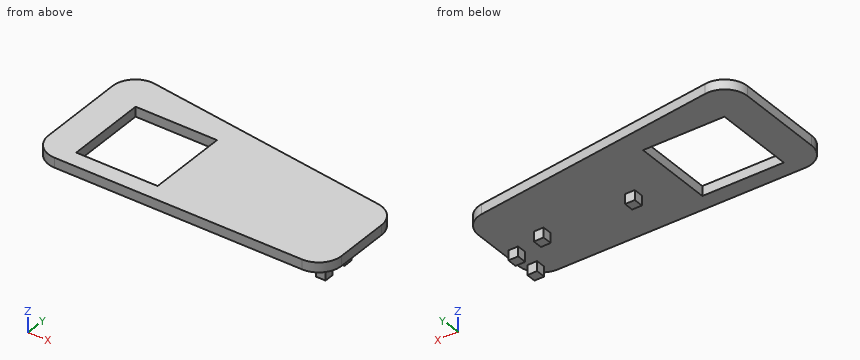
from build123d import *

# Parameters (mm, degrees)
PAD_DEPTH    = 3
SKETCH001_W  = 3
SKETCH001_H  = 3
PAD001_DEPTH = 3
FILLET_R     = 7
SKETCH002_W  = 25
SKETCH002_H  = 25
POCKET_DEPTH = 5


with BuildPart() as part:
    # Sketch → Pad (new body)
    with BuildSketch(Plane.XY):
        Polygon((0, 42), (0, 0), (90, 0), (90, 30), align=None)
    extrude(amount=PAD_DEPTH)

    # Sketch001 (on Face5 of Pad) → Pad001 (join)
    with BuildSketch(Plane(origin=(0, 0, 0), x_dir=(1, 0, 0), z_dir=(0, 0, -1))):
        with Locations((86.5, -4.5)):
            Rectangle(SKETCH001_W, SKETCH001_H)
        with Locations((86.5, -12.5)):
            Rectangle(SKETCH001_W, SKETCH001_H)
        with Locations((76.5, -15.5)):
            Rectangle(SKETCH001_W, SKETCH001_H)
        with Locations((48.5, -15.5)):
            Rectangle(SKETCH001_W, SKETCH001_H)
    extrude(amount=PAD001_DEPTH)

    # Fillet
    fillet_edges = [part.edges().sort_by_distance(p)[0] for p in [
        (0, 42, 1.5),
        (0, 0, 1.5),
        (90, 0, 1.5),
        (90, 30, 1.5),
    ]]
    fillet(fillet_edges, radius=FILLET_R)

    # Sketch002 (on Face2 of Fillet) → Pocket (cut)
    with BuildSketch(Plane(origin=(0, 0, 0), x_dir=(1, 0, 0), z_dir=(0, 0, -1))):
        with Locations((22.5, -17.5)):
            Rectangle(SKETCH002_W, SKETCH002_H)
    extrude(amount=-POCKET_DEPTH, mode=Mode.SUBTRACT)


solid = part.part
Read the model definition and answer for the solid it produces. Units are mm, in the model's axes. Coordinates: 2 decimals unless noted, no trailing zeros. Loops run counter-clockwise (first coordinate to the right, second up) from the corner with the lowest first, then second, coordinate; pieces in that order, holes last. Notation, with made-up numbers: (36, 83.25) - (67, 83.25) arc R21 cw to (67, 103.25) - close; hole circle Ø8 at (-14.5, 63.25). An arc over 180 degrees is marked (long way). Answer in a Markdown table with one row per item.
Q1. Given P1, Ø3.5, axis at x = 19, z = 2, coming from the +Y side; P2, Ø0.9, axis at y = 13, z = -1.5, coming from the +X side; P3, Ø0.9, axis at x = 48.5, z = -2, coming from the -Y side; P4, Ø10, axis at x = 20.5, y = 22, coming from the +Z side, each flat-ended and moving along its own axis, determine where each tip first touches the part or whether it passes through.
Here are the results:
| item | result |
|---|---|
| P1 | stops at y = 39.7 |
| P2 | stops at x = 88 |
| P3 | stops at y = 14 |
| P4 | passes through |
Q2. Find section C-C on x = 25. Write down the section's boundary in (y, z).
Here are the results:
| item | result |
|---|---|
| outline | (0, 0) - (5, 0) - (5, 3) - (0, 3) - close; (30, 0) - (38.67, 0) - (38.67, 3) - (30, 3) - close |
Q3. Find section B-B on y = 13. Write down the section's boundary in (x, z), plus the area to 3 significant figures.
Here are the results:
| item | result |
|---|---|
| outline | (0, 0) - (10, 0) - (10, 3) - (0, 3) - close; (35, 0) - (85, 0) - (85, -3) - (88, -3) - (88, 0) - (90, 0) - (90, 3) - (35, 3) - close |
| area | 204 mm^2 |
Q4. Find section A-A on z = 2. Write down the section's boundary in (x, y), plus the area to 3 significant figures.
Here are the results:
| item | result |
|---|---|
| outline | (0, 7) arc R7 ccw to (7, 0) - (83, 0) arc R7 ccw to (90, 7) - (90, 23.87) arc R7 ccw to (83.93, 30.81) - (7.93, 40.94) arc R7 ccw to (0, 34) - close; hole (10, 5) - (35, 5) - (35, 30) - (10, 30) - close |
| area | 2,570 mm^2 |
Q5. Find section D-D on x = 48. Write down the section's boundary in (y, z), plus the area to 3 significant figures.
Here are the results:
| item | result |
|---|---|
| outline | (0, 0) - (14, 0) - (14, -3) - (17, -3) - (17, 0) - (35.6, 0) - (35.6, 3) - (0, 3) - close |
| area | 116 mm^2 |
Q6. Straight lines are drawn through the part: line 1 along X through (y, z) = (15.5, -0.95); line 2 along X through (y, z) = (8.5, 0.65); line 3 along Z through (x, y) = (61.5, 4.5). For each, find the intervals that lie inside material, in ascending order. Write a range as [from, to].
Here are the results:
| item | result |
|---|---|
| line 1 | x = [47, 50], [75, 78] |
| line 2 | x = [0, 10], [35, 90] |
| line 3 | z = [0, 3] |
